from build123d import *

# Parameters (mm, degrees)
SKETCH1_W           = 8.4
SKETCH1_H           = 2.54
BOSS_EXTRUDE1_DEPTH = 2.54
CUT_EXTRUDE1_REACH  = 10.4
SKETCH2_W           = 0.74
SKETCH2_H           = 0.74
CHAMFER2_SIZE       = 0.8
CHAMFER2_SIZE2      = 1.2
SKETCH3_W           = 2.54
SKETCH3_H           = 0.54
CUT_EXTRUDE2_DEPTH  = 1
CUT_EXTRUDE4_START  = -6.2
SKETCH5_W           = 1.74
SKETCH5_H           = 0.54
CUT_EXTRUDE4_DEPTH  = 6.2


with BuildPart() as part:
    # Sketch1 → Boss-Extrude1 (new body)
    with BuildSketch(Plane.XY):
        with Locations((4.2, 1.27)):
            Rectangle(SKETCH1_W, SKETCH1_H)
    extrude(amount=BOSS_EXTRUDE1_DEPTH)

    # Sketch2 → Cut-Extrude1 (cut, up to next)
    with BuildSketch(Plane(origin=(8.4, 0, 0), x_dir=(0, 0, -1), z_dir=(1, 0, 0)), mode=Mode.PRIVATE) as cut_extrude1_sk1:
        with Locations((-1.27, 1.27)):
            Rectangle(SKETCH2_W, SKETCH2_H)
    cut_extrude1_tool1 = extrude(cut_extrude1_sk1.sketch, amount=-CUT_EXTRUDE1_REACH, mode=Mode.PRIVATE) & part.part
    add(cut_extrude1_tool1.solids().sort_by_distance((8.4, 1.27, 1.27))[0], mode=Mode.SUBTRACT)

    # Chamfer2
    chamfer2_edges = [part.edges().sort_by_distance(p)[0] for p in [
        (8.4, 1.27, 1.64),
        (8.4, 0.9, 1.27),
        (8.4, 1.27, 0.9),
        (8.4, 1.64, 1.27),
    ]]
    chamfer2_side = [part.faces().sort_by_distance(p)[0] for p in [
        (8.4, 0.035921024, 1.27),
    ]]
    chamfer(chamfer2_edges, length=CHAMFER2_SIZE, length2=CHAMFER2_SIZE2, reference=chamfer2_side[0])

    # Sketch3 → Cut-Extrude2 (cut)
    with BuildSketch(Plane.ZY):
        with Locations((1.27, 1.27)):
            Rectangle(SKETCH3_W, SKETCH3_H)
    extrude(amount=-CUT_EXTRUDE2_DEPTH, mode=Mode.SUBTRACT)

    # Sketch5 → Cut-Extrude4 (cut)
    with BuildSketch(Plane.ZY.offset(-1).offset(CUT_EXTRUDE4_START)):
        with Locations((1.27, 1.27)):
            Rectangle(SKETCH5_W, SKETCH5_H)
    extrude(amount=CUT_EXTRUDE4_DEPTH, mode=Mode.SUBTRACT)


solid = part.part
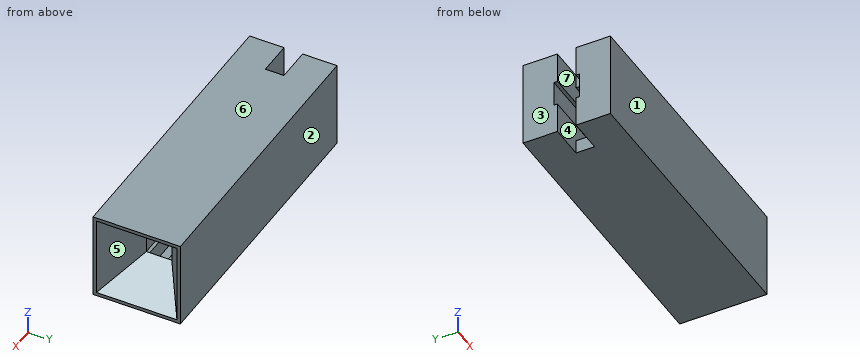
For this review, take the finished solid that the model builds, in its own axes (mm). Face numbers are marked on the shaded views. A direction names the side the tool comes from. Round coordinates to 2 decimals unless told otherwise and drop trailing zeros. Loops run counter-clockwise (first coordinate to the right, second up) from the corner with the lowest first, then second, coordinate; pieces in that order, holes last. Notation, with made-up numbers: (11.5, 58) - (40.5, 58) arc R19 ccw to (40.5, 63) - close; hole circle Ø1 at (-30.5, 41.5). An arc over 180 degrees is marked (long way). One line per item, written item: value. Start each with the question number.
Item 1: Take a section at C-C (y = 1.4). Give the boundary of the cut face in (x, z), plus the area to 3 significant figures.
Item 2: Take a section at A-A (z = 1.05). Give the boundary of the cut face in (x, y).
Item 3: The part is to be moulded in two halves that separate along Y. For the marked faces 1, 2, 3 and 4, say which applies: +Y half, -Y half, draft (parallel to the pull), parting line (faces both ways), or undercut.
Item 4: Take a section at B-B (x = 3.5). Give the boundary of the cut face in (y, z), plus the area to 3 significant figures.
Item 5: For L1, parallel to Y at x = 5.25, z = 1.7; L2, parallel to Y at x = 3, z = 1.1, list the stretches that pass through material, from the lowest coordinate up.
Item 6: For the marked faces 5, 6 and 7, list the 3-axis set-ups (+Z, -Z, +X, -X, +Y, -Y) from which the entire face can be reached by the end or side of a thin tool; tool diameter is ignored.
Item 7: Take a section at D-D (z = 2.3). Give the boundary of the cut face in (x, y).
Answer below:
1. outline: (1, 0) - (8.4, 0) - (8.4, 0.1) - (7.2, 0.9) - (7.2, 0.4) - (1, 0.4) - close; (1, 2.14) - (7.2, 2.14) - (7.2, 1.64) - (8.4, 2.44) - (8.4, 2.54) - (1, 2.54) - close
1. area: 6.16 mm2
2. outline: (0, 0) - (8.4, 0) - (8.4, 0.1) - (7.2, 0.9) - (0, 0.9) - close; (0, 1.64) - (7.2, 1.64) - (8.4, 2.44) - (8.4, 2.54) - (0, 2.54) - close
3. face 1: -Y half
3. face 2: +Y half
3. face 3: draft
3. face 4: undercut
4. outline: (0, 0) - (2.54, 0) - (2.54, 2.54) - (0, 2.54) - close; hole (0.9, 0.9) - (1, 0.9) - (1, 0.4) - (1.54, 0.4) - (1.54, 0.9) - (1.64, 0.9) - (1.64, 1.64) - (1.54, 1.64) - (1.54, 2.14) - (1, 2.14) - (1, 1.64) - (0.9, 1.64) - close
4. area: 5.36 mm2
5. L1: y = 0 to 1, 1.54 to 2.54
5. L2: y = 0 to 0.9, 1.64 to 2.54
6. face 5: +X
6. face 6: +Z, +X, -X, +Y, -Y
6. face 7: -X
7. outline: (0, 0) - (8.4, 0) - (8.4, 0.1) - (8.19, 0.24) - (8.19, 2.3) - (8.4, 2.44) - (8.4, 2.54) - (0, 2.54) - (0, 1.54) - (1, 1.54) - (1, 1) - (0, 1) - close
